```python
from build123d import *
from OCP.BRepAlgoAPI import BRepAlgoAPI_Cut
from OCP.TopTools import TopTools_ListOfShape

# Parameters (mm, degrees)
IZIM1_W                     = 45
IZIM1_H                     = 20
Y_KSEKLIK_EKSTR_ZYON1_DEPTH = 2
IZIM2_R                     = 3
IZIM2_R_2                   = 1
Y_KSEKLIK_EKSTR_ZYON2_DEPTH = 45
IZIM4_R                     = 1.5
KES_EKSTR_ZYON1_DEPTH       = 45
L_O_ALTMA1_COUNT            = 3
L_O_ALTMA1_PITCH            = 15
KES_EKSTR_ZYON3_START       = -11.25
KES_EKSTR_ZYON3_DEPTH       = 11.25
L_O_ALTMA7_START            = -11.25
L_O_ALTMA7_DEPTH            = 11.25


with BuildPart() as part:
    # Çizim1 → Yükseklik-Ekstrüzyon1 (new body)
    with BuildSketch(Plane(origin=(0, 0, 0), x_dir=(1, 0, 0), z_dir=(0, 1, 0))):
        Rectangle(IZIM1_W, IZIM1_H)
    extrude(amount=Y_KSEKLIK_EKSTR_ZYON1_DEPTH)

    # Çizim2 → Yükseklik-Ekstrüzyon2 (add)
    with BuildSketch(Plane(origin=(22.5, 0, 0), x_dir=(0, 0, -1), z_dir=(1, 0, 0))):
        with Locations((-9.996930096, 2.999998429)):
            Circle(IZIM2_R)
        with Locations((-9.996930096, 2.999998429)):
            Circle(IZIM2_R_2, mode=Mode.SUBTRACT)
    extrude(amount=-Y_KSEKLIK_EKSTR_ZYON2_DEPTH)

    # Çizim4 → Kes-Ekstrüzyon1 (cut)
    with BuildSketch(Plane(origin=(0, 2, 0), x_dir=(1, 0, 0), z_dir=(0, 1, 0))):
        with Locations(Location((-15, 1.415748792, 0), (0, 0, 270))):
            Circle(IZIM4_R)
    kes_ekstr_zyon1 = extrude(amount=-KES_EKSTR_ZYON1_DEPTH, mode=Mode.SUBTRACT)

    # LÇoğaltma1: Kes-Ekstrüzyon1 ×3
    with Locations(*[(i * L_O_ALTMA1_PITCH, 0, 0) for i in range(1, L_O_ALTMA1_COUNT)]):
        add(kes_ekstr_zyon1, mode=Mode.SUBTRACT)


with BuildPart() as kes_ekstr_zyon3_tool:
    # Kes-Ekstrüzyon3: read off the stored shape, not the designer's step
    # Kes-Ekstrüzyon3 outline → Kes-Ekstrüzyon3 (new body)
    with BuildSketch(Plane(origin=(22.5, 0, 0), x_dir=(0, 0, -1), z_dir=(1, 0, 0)).offset(KES_EKSTR_ZYON3_START)):
        with BuildLine():
            Line((-7.168502416, 0), (-7.168502416, 2))
            ThreePointArc((-7.168502416, 2), (-11.727728074, 5.450373576), (-10, 0))
            Line((-10, 0), (-7.168502416, 0))
        make_face()
        with BuildLine():
            Line((-9.996930096, 1.999998429), (-9.99999999, 2.000003141))
            ThreePointArc((-9.99999999, 2.000003141), (-9.995395236, 3.999997251), (-9.996930096, 1.999998429))
        make_face(mode=Mode.SUBTRACT)
    extrude(amount=KES_EKSTR_ZYON3_DEPTH)


with BuildPart() as part_1:
    add(part.part)

    # Kes-Ekstrüzyon3: cut by kes_ekstr_zyon3_tool, with a tolerance
    kes_ekstr_zyon3_stock = TopTools_ListOfShape()
    kes_ekstr_zyon3_stock.Append(part_1.part.wrapped)
    kes_ekstr_zyon3_tools = TopTools_ListOfShape()
    kes_ekstr_zyon3_tools.Append(kes_ekstr_zyon3_tool.part.wrapped)
    kes_ekstr_zyon3_cut = BRepAlgoAPI_Cut()
    kes_ekstr_zyon3_cut.SetArguments(kes_ekstr_zyon3_stock)
    kes_ekstr_zyon3_cut.SetTools(kes_ekstr_zyon3_tools)
    kes_ekstr_zyon3_cut.SetFuzzyValue(0.00001)
    kes_ekstr_zyon3_cut.Build()
    add(Compound.cast(kes_ekstr_zyon3_cut.Shape()).solids(), mode=Mode.REPLACE)


with BuildPart() as l_o_altma7_tool:
    # LÇoğaltma7: read off the stored shape, not the designer's step
    # LÇoğaltma7 outline → LÇoğaltma7 (new body)
    with BuildSketch(Plane.YZ.offset(L_O_ALTMA7_START)):
        with BuildLine():
            Line((0, 7.168502416), (2, 7.168502416))
            ThreePointArc((2, 7.168502416), (5.450373576, 11.727728074), (0, 10))
            Line((0, 10), (0, 7.168502416))
        make_face()
        with BuildLine():
            Line((1.999998429, 9.996930096), (2.000003141, 9.99999999))
            ThreePointArc((2.000003141, 9.99999999), (3.999997251, 9.995395236), (1.999998429, 9.996930096))
        make_face(mode=Mode.SUBTRACT)
    extrude(amount=L_O_ALTMA7_DEPTH)


with BuildPart() as part_2:
    add(part_1.part)

    # LÇoğaltma7: cut by l_o_altma7_tool, with a tolerance
    l_o_altma7_stock = TopTools_ListOfShape()
    l_o_altma7_stock.Append(part_2.part.wrapped)
    l_o_altma7_tools = TopTools_ListOfShape()
    l_o_altma7_tools.Append(l_o_altma7_tool.part.wrapped)
    l_o_altma7_cut = BRepAlgoAPI_Cut()
    l_o_altma7_cut.SetArguments(l_o_altma7_stock)
    l_o_altma7_cut.SetTools(l_o_altma7_tools)
    l_o_altma7_cut.SetFuzzyValue(0.00001)
    l_o_altma7_cut.Build()
    add(Compound.cast(l_o_altma7_cut.Shape()).solids(), mode=Mode.REPLACE)


solid = part_2.part
```
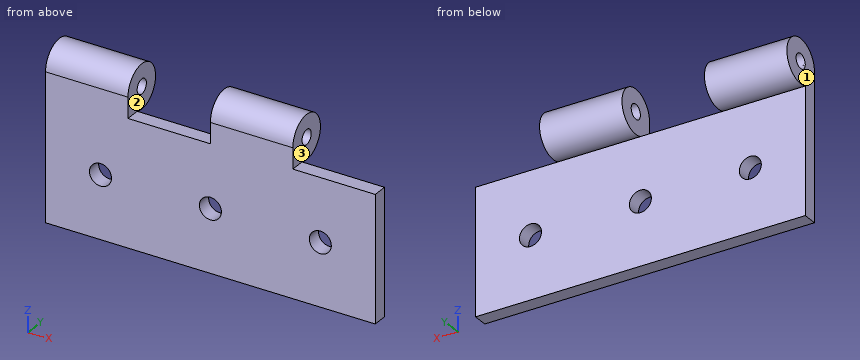
Input: part model. Units: mm. Frame: model coordinates. Face numbers are marked on the shaded views. Coordinates: 2 decimals unless noted, no trailing zeros. Loops run counter-clockwise (first coordinate to the right, second up) from the corner with the lowest first, then second, coordinate; pieces in that order, holes last. Notation, with made-up numbers: M -8,67.25 L -2,67.25 A12 cw -2,86.25 Z; hole C 83.5,5 d10. An arc over 180 degrees is marked long. Use a Markdown table: item, result. Add a question column.
1) Line query: L1, parallel to X at y = 3.25, z = 12; L2, parallel to Y at x = -3, z = -0.75; L3, parallel to Z at x = 20.5, y = 0.5. Output: solid intervals per line, ascending. Write a range as from..to.
2) Section D-D, the plane z = 11.5. Return the cut outline in (x, y), plus the area to 3 significant figures.
3) Section B-B, the plane x = 15. Return the cut outline in (y, z), plus the area to 3 significant figures.
4) Section C-C, the plane y = 3. Return the cut outline in (x, z), plus the area to 3 significant figures.
5) Draft query along X for the marked faces 1, 2 and 3. Return one class per face: +X half, -X half, draft (parallel to the pull), parting line (faces both ways), or undercut.
6) Pin query (flat end, axial travel): P1, Ø1.8, axis at x = -15, z = -1.42, coming from the +Y side (3 decimals); P2, Ø2, axis at y = 4, z = 6.5, coming from the +X side; P3, Ø1, axis at x = -6.5, y = 1, coming from the +Z side; P4, Ø5, axis at x = 7.5, z = 0.5, coming from the +Y side. Return the tip coordinate at first contact, or that it passes through.
7) Section A-A, the plane x = -15. Give the number of separate pieces and of enclosed holes in the cut face, plus the area to 3 significant figures.
Answer below:
| question | item | result |
|---|---|---|
| 1 | L1 | -22.5..-11.25, 0..11.25 |
| 1 | L2 | 0..2 |
| 1 | L3 | -10..7.17 |
| 2 | outline | M -22.5,0.4 L -11.25,0.4 L -11.25,5.6 L -22.5,5.6 Z; M 0,0.4 L 11.25,0.4 L 11.25,5.6 L 0,5.6 Z |
| 2 | area | 117 mm2 |
| 3 | outline | M 0,-10 L 2,-10 L 2,-2.92 L 0,-2.92 Z; M 0,0.08 L 2,0.08 L 2,7.17 L 0,7.17 Z |
| 3 | area | 28.3 mm2 |
| 4 | outline | M -22.5,7 L -11.25,7 L -11.25,9 L -22.5,9 Z; M -22.5,11 L -11.25,11 L -11.25,13 L -22.5,13 Z; M 0,7 L 11.25,7 L 11.25,9 L 0,9 Z; M 0,11 L 11.25,11 L 11.25,13 L 0,13 Z |
| 4 | area | 90.0 mm2 |
| 5 | face 1 | -X half |
| 5 | face 2 | undercut |
| 5 | face 3 | +X half |
| 6 | P1 | through |
| 6 | P2 | x = 11.25 |
| 6 | P3 | z = 7.17 |
| 6 | P4 | y = 2 |
| 7 | separate pieces | 2 |
| 7 | enclosed holes | 1 |
| 7 | area | 55.0 mm2 |
